Can you work these out from the model? Positions are in its coordinate system, mm. A direction names the side the tool comes from. Give positions to 0.01 mm unless a question says otherwise; leave off trailing zeros. Order: outer loops, then holes, each group sorted by start corner. A loop starts at its lowest first (then second) coordinate and runs counter-clockwise, first axis right, second up. Notation, with made-up numbers: (14.25, 22) - (46.25, 22) arc R20 cw to (46.25, 54) - close; hole circle Ø6 at (85.5, 29). An arc over 180 degrees is marked (long way). Answer as CSV lines item,"result".
```python
from build123d import *

# Parameters (mm, degrees)
F0_R     = 7
F0_R_2   = 2.5
F1_DEPTH = 2.5
F2_R     = 6.298938
F2_R_2   = 3.223977
F3_DEPTH = 0.25
F4_R     = 0.25


with BuildPart() as f1:
    # F0 (on Top) → F1 (new body)
    with BuildSketch(Plane.XY):
        Circle(F0_R)
        Circle(F0_R_2, mode=Mode.SUBTRACT)
    extrude(amount=F1_DEPTH)

    # F2 (on face) → F3 (cut)
    with BuildSketch(Plane.XY.offset(2.5)):
        Circle(F2_R)
        Circle(F2_R_2, mode=Mode.SUBTRACT)
    extrude(amount=-F3_DEPTH, mode=Mode.SUBTRACT)

    # F4
    f4_edges = [f1.edges().sort_by_distance(p)[0] for p in [
        (-7, 0, 2.5),
        (-2.5, 0, 2.5),
    ]]
    fillet(f4_edges, radius=F4_R)

    # F5: F1 across face


with BuildPart() as f1_1:
    add(f1.part)
    add(f1.part.mirror(Plane(origin=(0, 0, 0), x_dir=(1, 0, 0), z_dir=(0, 0, -1))))


solid = f1_1.part
```
1) If we mould it in two halves opening along X, with no side actions, what happens to faces 1 (the flat face through (3, -3, -2.25)), 2 (the cylindrical face through (6.466, -2.681, 0.031))? For each: +X half, -X half, draft (parallel to the pull), parting line (faces both ways), or undercut.
Answer block:
face 1,"undercut"
face 2,"parting line"
2) I'm going to push flat-ended pins straight in: P1, Ø4, axis at x = -0.5, y = -0.5, coming from the -Z side; P2, Ø1, axis at x = -1, z = 0.5, coming from the -Y side; P3, Ø4.5, axis at x = 0, y = 0, coming from the +Z side. Where does each tip first touch, or does it pass through?
Answer block:
P1,"z = -2.5"
P2,"y = -6.98"
P3,"through"
3) I need wall thicknesses on line 1 along Y through (x, z) = (0, -0.85); line 2 along Y through (x, z) = (0, -2.35); line 3 along Z through (x, y) = (1.75, 3.75). Which ranges of each line are inside material? Lowest first, please. Write a range as [from, to].
Answer block:
line 1,"[-7, -2.5], [2.5, 7]"
line 2,"[-6.98, -6.3], [-3.22, -2.52], [2.52, 3.22], [6.3, 6.98]"
line 3,"[-2.25, 2.25]"
4) Which directions (+Z, -Z, +X, -X, +Y, -Y) give clear straight access to the entire face, cutting with the end or side of a thin tool? Please do faces 3 (the cylindrical face through (-0.54, -2.44, -0.03)), 4 (the flat face through (3, -3, 2.25)).
Answer block:
face 3,"+Z, -Z"
face 4,"+Z"
5) I want a section at C-C on z = 0.95. Write out the boundary of the cut face in (x, y), plus the area to 3 significant figures.
Answer block:
outline,"circle Ø14 at (0, 0); hole circle Ø5 at (0, 0)"
area,"134 mm2"
